Verification items for the finished model (mm, model axes). Face numbers are marked on the shaded views. A direction names the side the tool comes from. Round coordinates to 2 decimals unless told otherwise and drop trailing zeros. Order: outer loops, then holes, each group sorted by start corner. A loop starts at its lowest first (then second) coordinate and runs counter-clockwise, first axis right, second up. Notation, with made-up numbers: (-31.75, 32) -> (23.25, 32) arc R25 cw to (23.25, 55) -> close; hole circle Ø3 at (12.5, -15). An arc over 180 degrees is marked (long way). Put each result on its own line as item: value.
Autodesk Inventor part; units mm, degrees
ref_plane "YZ Plane" through (0, 0, 0) normal (1, 0, 0) x (0, 1, 0)
ref_plane "XZ Plane" through (0, 0, 0) normal (0, 1, 0) x (-1, 0, 0)
ref_plane "XY Plane" through (0, 0, 0) normal (0, 0, 1) x (1, 0, 0)
sketch "Sketch1" plane through (0, 0, 0) normal (0, 1, 0) x (-1, 0, 0)
  circle A0 centre (0, 0) radius 3.9878
  dimension "d0" = 7.9756
extrude "Extrusion1" add sketch "Sketch1" along normal blind 0.3302
sketch "Sketch2" plane through (0, 0.3302, 0) normal (0, 1, 0) x (1, 0, 0)
  circle A0 centre (0, 0) radius 3.9878
  arc A1 (-3.9382, 0.627) -> (-3.9382, -0.627) centre (0, 0) ccw
  line L0 (-3.9382, -0.627) -> (-3.9382, 0.627) construction
  line L1 (-3.9382, -0.627) -> (-2.6841, -0.627) construction
  line L2 (-3.9382, -0.627) -> (-3.8546, -0.6035)
  line L3 (-3.9382, 0.627) -> (-3.8546, 0.6111)
  line L4 (-3.8546, 0.6111) -> (-3.8546, -0.6035)
  line L5 (-2.4566, -3.0327) -> (-1.4047, -3.64)
  arc A2 (-2.5121, -3.0971) -> (-1.4261, -3.7241) centre (0, 0) ccw
  line L6 (-1.4261, -3.7241) -> (-1.4047, -3.64)
  line L7 (-2.5121, -3.0971) -> (-2.4566, -3.0327)
  line L8 (1.3981, -3.6438) -> (2.45, -3.0365)
  arc A3 (1.4261, -3.7241) -> (2.5121, -3.0971) centre (0, 0) ccw
  line L9 (2.5121, -3.0971) -> (2.45, -3.0365)
  line L10 (1.4261, -3.7241) -> (1.3981, -3.6438)
  line L11 (3.8546, -0.6111) -> (3.8546, 0.6035)
  arc A4 (3.9382, -0.627) -> (3.9382, 0.627) centre (0, 0) ccw
  line L12 (3.9382, 0.627) -> (3.8546, 0.6035)
  line L13 (3.9382, -0.627) -> (3.8546, -0.6111)
  line L14 (2.4566, 3.0327) -> (1.4047, 3.64)
  arc A5 (2.5121, 3.0971) -> (1.4261, 3.7241) centre (0, 0) ccw
  line L15 (1.4261, 3.7241) -> (1.4047, 3.64)
  line L16 (2.5121, 3.0971) -> (2.4566, 3.0327)
  line L17 (-1.3981, 3.6438) -> (-2.45, 3.0365)
  arc A6 (-1.4261, 3.7241) -> (-2.5121, 3.0971) centre (0, 0) ccw
  line L18 (-2.5121, 3.0971) -> (-2.45, 3.0365)
  line L19 (-1.4261, 3.7241) -> (-1.3981, 3.6438)
  dimension "d3" = 90
  dimension "d6" = 360
extrude "Extrusion2" add sketch "Sketch2" along normal blind 7.9248 contours A0 L13 L11 L12 | L16 L14 L15 A0 | A0 L10 L8 L9 | L19 L17 L18 A0 | A0 L7 L5 L6 | L3 L4 L2 A0
fillet "Fillet1" radius 0.1905 1 edges at (3.9878, 0, 0)
sketch "Sketch3" plane through (0, 0.3302, 0) normal (0, 1, 0) x (1, 0, 0)
  line L0 (-0.9525, 1.016) -> (-1.2827, 1.016)
  line L1 (-1.2827, 1.016) -> (-1.2827, -1.016)
  line L2 (-1.2827, -1.016) -> (-0.9525, -1.016)
  line L3 (-0.9525, -1.016) -> (-0.9525, 1.016)
  line L4 (0, 2.5556) -> (0, -1.5997)
  line L5 (0.9525, 1.016) -> (1.2827, 1.016)
  line L6 (1.2827, 1.016) -> (1.2827, -1.016)
  line L7 (1.2827, -1.016) -> (0.9525, -1.016)
  line L8 (0.9525, -1.016) -> (0.9525, 1.016)
  point P0 (0, 0)
  dimension "d11" = 0.3302
  dimension "d12" = 2.032
  dimension "d13" = 1.016
  dimension "d14" = 0.9525
extrude "Extrusion3" add sketch "Sketch3" along normal blind 9.525
sketch "Sketch5" plane through (1.2827, 0.3302, 1.016) normal (1, 0, 0) x (0, 0, -1)
  circle A0 centre (1.016, 9.0059) radius 0.9525
  point P0 (1.016, -0.3302)
  dimension "d18" = 1.905
extrude "Extrusion4" cut sketch "Sketch5" against normal through all
properties part number "piston holder thing" material "Aluminum 6061"
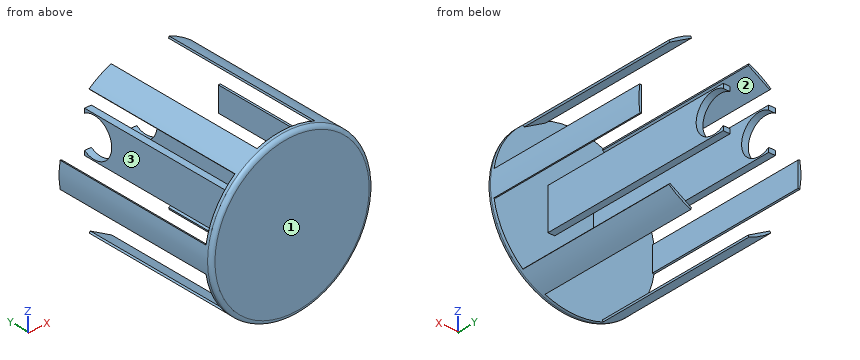
Item 1: Sectioned sample at C-C, the plane y = 9.25. Record the boundary of the cut face in (x, z), then the cut area to 3 significant figures.
Geometry check:
outline: (-1.28, -1.02) -> (-0.95, -1.02) -> (-0.95, -0.95) -> (-1.28, -0.95) -> close; (-1.28, 0.95) -> (-0.95, 0.95) -> (-0.95, 1.02) -> (-1.28, 1.02) -> close; (0.95, -1.02) -> (1.28, -1.02) -> (1.28, -0.95) -> (0.95, -0.95) -> close; (0.95, 0.95) -> (1.28, 0.95) -> (1.28, 1.02) -> (0.95, 1.02) -> close
area: 0.0890 mm2
Item 2: Tool access check on the marked faces 1, 2 and 3. Record the directions out of +Z, -Z, +X, -X, +Y, -Y that give a thin tool (end or side, any length) a straight path to the whole face; none if there is none.
Geometry check:
face 1: +Z, -Z, +X, -X, -Y
face 2: +Y
face 3: +Z, -Z, +Y
Item 3: Material ranges on line 1 along X through (y, z) = (7.5, 0.75); line 2 along Y through (x, z) = (-3, 2); line 3 along Z through (x, y) = (1, 1.5), recorded low to high.
Geometry check:
line 1: -1.28 to -0.95, 0.95 to 1.28
line 2: 0 to 0.33
line 3: -1.02 to 1.02
Item 4: Sectioned sample at A-A, the plane y = 1. Give the number of separate pieces and of enclosed holes in the cut face, then the cut area to 3 significant figures.
Geometry check:
separate pieces: 8
enclosed holes: 0
area: 2.21 mm2
Item 5: Sectioned sample at B-B, the plane x = 0. Record the boundary of the cut face in (y, z), then the cut area to 3 significant figures.
Geometry check:
outline: (0, -3.8) arc R0.19 ccw to (0.19, -3.99) -> (0.33, -3.99) -> (0.33, 3.99) -> (0.19, 3.99) arc R0.19 ccw to (0, 3.8) -> close
area: 2.62 mm2
Item 6: Depth check by flat-ended pin: pin 1 Ø1.6 at (y, z) = (3.5, -0.5) entering from +X; pin 2 Ø3 at (x, y) = (-0.5, 3.5) entering from -Z; pin 3 Ø0.6 at (y, z) = (4, 0.5) entering from -X; pin 4 Ø2 at (x, y) = (3, 2) entering from -Z. Enter the tip coordinate at first touch or a pass-through.
Geometry check:
pin 1: x = 3.99
pin 2: z = -3.72
pin 3: x = -3.98
pin 4: z = -3.45
